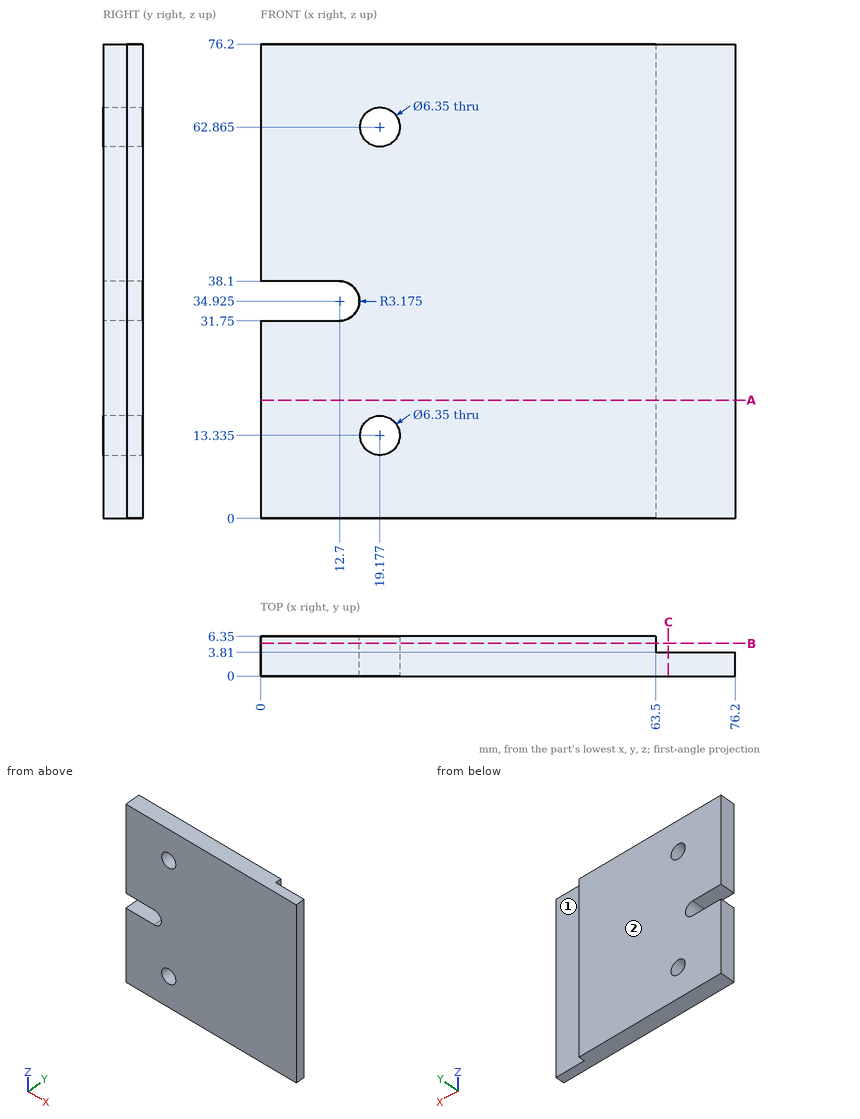
Source: three-view drawing plus pictorial views. Frame: mm from the lowest corner of the part. A direction names the side the tool comes from. Coordinates: 2 decimals unless noted, no trailing zeros. Order: outer loops, then holes, each group sorted by start corner. A loop starts at its lowest first (then second) coordinate and runs counter-clockwise, first axis right, second up. Notation, with made-up numbers: M 55,-2 L 81,-2 A26 ccw 81,20 Z; hole C 42,-17.5 d11. An arc over 180 degrees is marked long. One line per question, with ' | ' between items. Start each with the question number.
Item 1: Set-up query: the marked faces 1 and 2. Return all of +Z, -Z, +X, -X, +Y, -Y with unobstructed straight access to the full face (end or side cutting, diameter ignored); none if empty.
Item 2: Cut plane A-A, the plane z = 19. Return the cut outline in (x, y), then the cut area to 3 significant figures.
Item 3: Cut plane C-C, the plane x = 65.5. Return the cut outline in (y, z).
Item 4: Pin query (flat end, axial travel): pin 1 Ø4 at (x, z) = (16, 11.5) entering from -Y; pin 2 Ø1.3 at (y, z) = (4.5, 26.5) entering from +X; pin 3 Ø6.5 at (x, z) = (69.5, 44.5) entering from +Y; pin 4 Ø5.5 at (x, z) = (19.177, 62.865) entering from +Y. Return the tip coordinate at first contact, or that it passes through.
Item 5: Ray query, probe 1 along Z at (x, y) = (10, 1.5); probe 2 along X at (y, z) = (4.5, 57); probe 3 along Y at (x, z) = (72.5, 23). Return the intervals inside material, ascending. Write a range as [from, to].
Item 6: Cut plane B-B, the plane y = 5.25. Return the cut outline in (x, z) (3 decimals), then the cut area to 3 significant figures.
A:
1) face 1: +Z, -Z, +X, +Y | face 2: +Z, -Z, +X, -X, +Y
2) outline: M 0,0 L 76.2,0 L 76.2,3.81 L 63.5,3.81 L 63.5,6.35 L 0,6.35 Z | area: 452 mm2
3) outline: M 0,0 L 3.81,0 L 3.81,76.2 L 0,76.2 Z
4) pin 1: stops at y = 0 | pin 2: stops at x = 63.5 | pin 3: stops at y = 3.81 | pin 4: passes through
5) probe 1: z = [0, 31.75], [38.1, 76.2] | probe 2: x = [0, 63.5] | probe 3: y = [0, 3.81]
6) outline: M 0,0 L 63.5,0 L 63.5,76.2 L 0,76.2 L 0,38.1 L 12.7,38.1 A3.175 cw 12.7,31.75 L 0,31.75 Z; hole C 19.177,13.335 d6.35; hole C 19.177,62.865 d6.35 | area: 4,680 mm2
